Verification items for the finished model (mm, model axes). Face numbers are marked on the shaded views. A direction names the side the tool comes from. Coordinates: 2 decimals unless noted, no trailing zeros. Write each loop counter-clockwise with the first axis right and the second up, starting at its lowest first coordinate (ties: lowest second). Pieces come first, ordered by that corner, then holes.
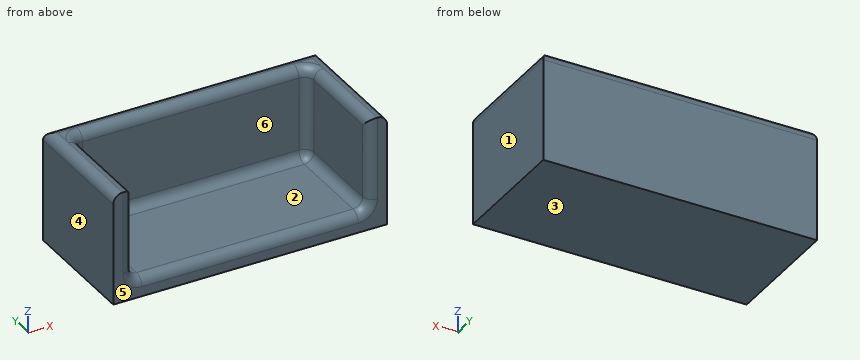
```python
from build123d import *

# Parameters (mm, degrees)
F0_W     = 2184.4
F0_H     = 990.6
F1_DEPTH = 889
F2_T     = -152.4
F3_R     = 76.2
F4_R     = 76.19999


# Not quite as in the source:
# - a fillet or chamfer is up to 0.001 mm smaller than in the source, because OpenCascade refuses the exact size


with BuildPart() as f1:
    # F0 (on Top) → F1 (new body)
    with BuildSketch(Plane.XY):
        with Locations((2.5491379201, 53.3265618357)):
            Rectangle(F0_W, F0_H)
    extrude(amount=F1_DEPTH)

    # F2
    f2_openings = [f1.faces().sort_by_distance(p)[0] for p in [
        (2.549138, 53.326562, 889),
        (2.549138, -441.973438, 444.5),
    ]]
    offset(amount=F2_T, openings=f2_openings)

    # F3
    f3_edges = [f1.edges().sort_by_distance(p)[0] for p in [
        (2.549138, 396.226562, 889),
        (-937.250862, 396.226562, 520.7),
        (2.549138, 396.226562, 152.4),
        (942.349138, 396.226562, 520.7),
        (2.549138, -441.973438, 152.4),
        (942.349138, -22.873438, 152.4),
        (-937.250862, -22.873438, 152.4),
        (-937.250862, -441.973438, 520.7),
        (-937.250862, -22.873438, 889),
        (942.349138, -441.973438, 520.7),
        (942.349138, -22.873438, 889),
    ]]
    fillet(f3_edges, radius=F3_R)

    # F4 (radius 76.2 in the source; OpenCascade refuses exactly that, so slightly less here)
    f4_edges = [f1.edges().sort_by_distance(p)[0] for p in [
        (1094.749138, 53.326562, 889),
        (2.549138, 548.626562, 889),
        (-1089.650862, 53.326562, 889),
    ]]
    fillet(f4_edges, radius=F4_R)


solid = f1.part
```
1. Gauge pin test, flat ends, axial feed: P1, Ø6, axis at x = 870.5, y = 132, coming from the +Z side; P2, Ø8, axis at x = -633, y = 374.5, coming from the +Z side. Record the tip position at first contact, or that the pin passes through.
2. Tool access check on the marked faces 5 and 6. Record the directions out of +Z, -Z, +X, -X, +Y, -Y that give a thin tool (end or side, any length) a straight path to the whole face; none if there is none.
3. Material ranges on L1, parallel to X at y = -297, z = 489; L2, parallel to Z at x = 835.5, y = 208.5; L3, parallel to Y at x = 223.5, z = 289.5, recorded low to high.
4. Sectioned sample at A-A, the plane z = 525. Record the boundary of the cut face in (x, y), and give its area (3 significant figures).
5. Draft check along X on the marked faces 1, 2, 3 and 4. Enter one of: pulls with the +X half, pulls with the -X half, needs draft (parallel to the pull), parting line crosses it, or undercut.
Outcome:
1. P1: stops at z = 152.76
1. P2: stops at z = 179.74
2. face 5: +Z, -Z, +X, -X, -Y
2. face 6: +Z, -Y
3. L1: x = -1089.65 to -937.25, 942.35 to 1094.75
3. L2: z = 0 to 152.4
3. L3: y = 396.23 to 548.63
4. outline: (-1089.65, -441.97) - (-1013.45, -441.97) arc R76.2 ccw to (-937.25, -365.77) - (-937.25, 320.03) arc R76.2 cw to (-861.05, 396.23) - (866.15, 396.23) arc R76.2 cw to (942.35, 320.03) - (942.35, -365.77) arc R76.2 ccw to (1018.55, -441.97) - (1094.75, -441.97) - (1094.75, 548.63) - (-1089.65, 548.63) - close
4. area: 588,000 mm2
5. face 1: pulls with the +X half
5. face 2: undercut
5. face 3: needs draft
5. face 4: pulls with the -X half
